Verification items for the finished model (mm, model axes). Face numbers are marked on the shaded views. Round coordinates to 2 decimals unless told otherwise and drop trailing zeros. Write each loop counter-clockwise with the first axis right and the second up, starting at its lowest first coordinate (ties: lowest second). Pieces come first, ordered by that corner, then holes. Notation, with made-up numbers: M 84.25,79.25 L 111.25,79.25 A7 ccw 111.25,90.25 Z; hole C 83.25,77 d3. An arc over 180 degrees is marked long. Answer in a Markdown table with one row per item. Add a question column.
1. Sectioned sample at C-C on z = 8.5. Record the cut outline in (x, y).
2. Material ranges on probe 1 along Z at (x, y) = (4, 0); probe 2 along Z at (x, y) = (13.3, 0); probe 3 along X at (y, z) = (-2.5, 30), recorded low to high.
3. Sectioned sample at B-B on y = 0. Record the cut outline in (x, z), plus the area to 3 significant figures.
4. Sectioned sample at D-D on x = -14.5. Record the cut outline in (y, z).
5. Sectioned sample at A-A on z = 36. Record the cut outline in (x, y) (3 decimals), plus the area to 3 significant figures.
6. Draft check along X on the marked faces 1, 2 and 3. Enter one of: pulls with the +X half, pulls with the -X half, needs draft (parallel to the pull), parting line crosses it, or undercut.
7. Go/stop test with flat-tipped pins: pin 1 Ø1 at (x, z) = (10.5, 9) entering from -Y; pin 2 Ø4.5 at (y, z) = (0, 20.15) entering from +X; pin 3 Ø1.2 at (x, z) = (6, 34.5) entering from -Y. Record where each tip stops, or that it passes through.
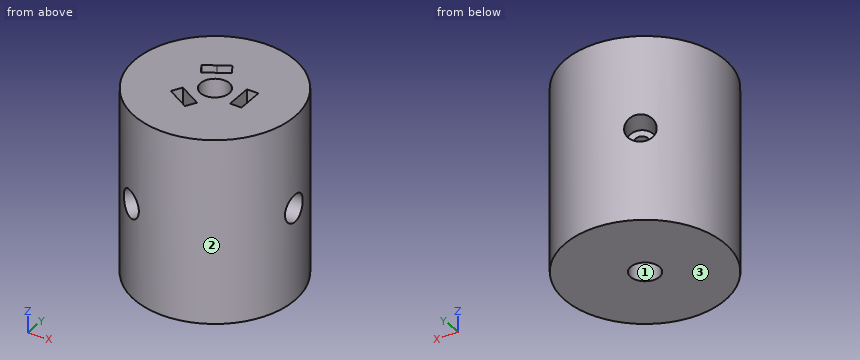
```python
from build123d import *

# Parameters (mm, degrees)
SKETCH1_R           = 17.5
SKETCH1_R_2         = 3.15
BOSS_EXTRUDE1_DEPTH = 40.3
CUT_EXTRUDE1_DEPTH  = 23
CUT_EXTRUDE4_REACH  = 43.405
SKETCH8_R           = 1.65
CUT_EXTRUDE5_REACH  = 43.405
SKETCH10_R          = 1.65
SKETCH12_R          = 3
CUT_EXTRUDE6_DEPTH  = 5.35
SKETCH15_R          = 3
CUT_EXTRUDE8_DEPTH  = 5.35
CUT_EXTRUDE9_REACH  = 43.405
SKETCH17_R          = 1.65
CUT_EXTRUDE10_REACH = 43.405
SKETCH18_R          = 1.65
SKETCH19_R          = 3
CUT_EXTRUDE11_DEPTH = 5.35
CUT_EXTRUDE12_REACH = 37
SKETCH20_R          = 1.65
CUT_EXTRUDE13_REACH = 37
SKETCH21_R          = 1.65


with BuildPart() as part:
    # Sketch1 → Boss-Extrude1 (new body)
    with BuildSketch(Plane.XY):
        Circle(SKETCH1_R)
        Circle(SKETCH1_R_2, mode=Mode.SUBTRACT)
    extrude(amount=BOSS_EXTRUDE1_DEPTH)

    # Sketch2 → Cut-Extrude1 (cut)
    with BuildSketch(Plane.XY.offset(40.3)):
        Polygon((7.65, 0), (7.65, 2.85), (5.15, 2.85), (5.15, -2.85), (7.65, -2.85), align=None)
        Polygon((-3.825, -6.625094339), (-1.356827599, -8.050094339), (-0.106827599, -5.885030829), (-5.043172401, -3.035030829), (-6.293172401, -5.200094339), align=None)
        Polygon((-3.825, 6.625094339), (-6.293172401, 5.200094339), (-5.048242412, 3.035349353), (-0.105426694, 5.882604512), (-1.356827546, 8.050094369), align=None)
    extrude(amount=-CUT_EXTRUDE1_DEPTH, mode=Mode.SUBTRACT)

    # Sketch8 → Cut-Extrude4 (cut, up to next)
    with BuildSketch(Plane(origin=(-8.75, -15.155444566, 0), x_dir=(0, 0, -1), z_dir=(-0.5, -0.866025404, 0)), mode=Mode.PRIVATE) as cut_extrude4_sk1:
        with Locations((-20.15, 0)):
            Circle(SKETCH8_R)
    cut_extrude4_tool1 = extrude(cut_extrude4_sk1.sketch, amount=-CUT_EXTRUDE4_REACH, mode=Mode.PRIVATE) & part.part
    add(cut_extrude4_tool1.solids().sort_by_distance((-8.75, -15.155445, 20.15))[0], mode=Mode.SUBTRACT)

    # Sketch10 → Cut-Extrude5 (cut, up to next)
    with BuildSketch(Plane(origin=(-8.75, -15.155444566, 0), x_dir=(0, 0, -1), z_dir=(-0.5, -0.866025404, 0)), mode=Mode.PRIVATE) as cut_extrude5_sk1:
        with Locations((-20.15, 0)):
            Circle(SKETCH10_R)
    cut_extrude5_tool1 = extrude(cut_extrude5_sk1.sketch, amount=-CUT_EXTRUDE5_REACH, mode=Mode.PRIVATE) & part.part
    add(cut_extrude5_tool1.solids().sort_by_distance((-8.75, -15.155445, 20.15))[0], mode=Mode.SUBTRACT)

    # Sketch12 → Cut-Extrude6 (cut)
    with BuildSketch(Plane(origin=(-8.75, -15.155444566, 0), x_dir=(0, 0, -1), z_dir=(-0.5, -0.866025404, 0))):
        with Locations((-20.15, 0)):
            Circle(SKETCH12_R)
    extrude(amount=-CUT_EXTRUDE6_DEPTH, mode=Mode.SUBTRACT)

    # Sketch15 → Cut-Extrude8 (cut)
    with BuildSketch(Plane(origin=(-8.75, 15.155444566, 0), x_dir=(0, 0, -1), z_dir=(-0.5, 0.866025404, 0))):
        with Locations((-20.15, 0)):
            Circle(SKETCH15_R)
    extrude(amount=-CUT_EXTRUDE8_DEPTH, mode=Mode.SUBTRACT)

    # Sketch17 → Cut-Extrude9 (cut, up to next)
    with BuildSketch(Plane(origin=(-8.75, 15.155444566, 0), x_dir=(0, 0, -1), z_dir=(-0.5, 0.866025404, 0)), mode=Mode.PRIVATE) as cut_extrude9_sk1:
        with Locations((-20.15, 0)):
            Circle(SKETCH17_R)
    cut_extrude9_tool1 = extrude(cut_extrude9_sk1.sketch, amount=-CUT_EXTRUDE9_REACH, mode=Mode.PRIVATE) & part.part
    add(cut_extrude9_tool1.solids().sort_by_distance((-8.75, 15.155445, 20.15))[0], mode=Mode.SUBTRACT)

    # Sketch18 → Cut-Extrude10 (cut, up to next)
    with BuildSketch(Plane(origin=(-8.75, 15.155444566, 0), x_dir=(0, 0, -1), z_dir=(-0.5, 0.866025404, 0)), mode=Mode.PRIVATE) as cut_extrude10_sk1:
        with Locations((-20.15, 0)):
            Circle(SKETCH18_R)
    cut_extrude10_tool1 = extrude(cut_extrude10_sk1.sketch, amount=-CUT_EXTRUDE10_REACH, mode=Mode.PRIVATE) & part.part
    add(cut_extrude10_tool1.solids().sort_by_distance((-8.75, 15.155445, 20.15))[0], mode=Mode.SUBTRACT)

    # Sketch19 → Cut-Extrude11 (cut)
    with BuildSketch(Plane(origin=(17.5, 0, 0), x_dir=(0, 0, -1), z_dir=(1, 0, 0))):
        with Locations((-20.15, 0)):
            Circle(SKETCH19_R)
    extrude(amount=-CUT_EXTRUDE11_DEPTH, mode=Mode.SUBTRACT)

    # Sketch20 → Cut-Extrude12 (cut, up to next)
    with BuildSketch(Plane(origin=(17.5, 0, 0), x_dir=(0, 0, -1), z_dir=(1, 0, 0)), mode=Mode.PRIVATE) as cut_extrude12_sk1:
        with Locations((-20.15, 0)):
            Circle(SKETCH20_R)
    cut_extrude12_tool1 = extrude(cut_extrude12_sk1.sketch, amount=-CUT_EXTRUDE12_REACH, mode=Mode.PRIVATE) & part.part
    add(cut_extrude12_tool1.solids().sort_by_distance((17.5, 0, 20.15))[0], mode=Mode.SUBTRACT)

    # Sketch21 → Cut-Extrude13 (cut, up to next)
    with BuildSketch(Plane(origin=(17.5, 0, 0), x_dir=(0, 0, -1), z_dir=(1, 0, 0)), mode=Mode.PRIVATE) as cut_extrude13_sk1:
        with Locations((-20.15, 0)):
            Circle(SKETCH21_R)
    cut_extrude13_tool1 = extrude(cut_extrude13_sk1.sketch, amount=-CUT_EXTRUDE13_REACH, mode=Mode.PRIVATE) & part.part
    add(cut_extrude13_tool1.solids().sort_by_distance((17.5, 0, 20.15))[0], mode=Mode.SUBTRACT)


solid = part.part
```
Geometry check:
| question | item | result |
|---|---|---|
| 1 | outline | C 0,0 d35; hole C 0,0 d6.3 |
| 2 | probe 1 | z = 0 to 18.5, 21.8 to 40.3 |
| 2 | probe 2 | z = 0 to 17.15, 23.15 to 40.3 |
| 2 | probe 3 | x = -17.32 to -1.92, 1.92 to 5.15, 7.65 to 17.32 |
| 3 | outline | M -17.5,0 L -3.15,0 L -3.15,40.3 L -17.5,40.3 Z; M 3.15,0 L 17.5,0 L 17.5,17.15 L 12.15,17.15 L 12.15,18.5 L 7.65,18.5 L 7.65,17.3 L 5.15,17.3 L 5.15,18.5 L 3.15,18.5 Z; M 3.15,21.8 L 5.15,21.8 L 5.15,40.3 L 3.15,40.3 Z; M 7.65,21.8 L 12.15,21.8 L 12.15,23.15 L 17.5,23.15 L 17.5,40.3 L 7.65,40.3 Z |
| 3 | area | 1,050 mm2 |
| 4 | outline | M -9.8,0 L 9.8,0 L 9.8,40.3 L -9.8,40.3 Z |
| 5 | outline | C 0,0 d35; hole M -6.293,-5.2 L -1.357,-8.05 L -0.107,-5.885 L -5.043,-3.035 Z; hole M -6.293,5.2 L -5.048,3.035 L -0.105,5.883 L -1.357,8.05 Z; hole C 0,0 d6.3; hole M 5.15,-2.85 L 7.65,-2.85 L 7.65,2.85 L 5.15,2.85 Z |
| 5 | area | 888 mm2 |
| 6 | face 1 | undercut |
| 6 | face 2 | parting line crosses it |
| 6 | face 3 | needs draft |
| 7 | pin 1 | stops at y = -14.36 |
| 7 | pin 2 | stops at x = 12.15 |
| 7 | pin 3 | stops at y = -16.65 |
